The listing builds one solid part. Answer for the finished solid, in the listing's coordinates (mm). Face numbers are marked on the shaded views. A direction names the side the tool comes from. Give positions to 0.01 mm unless a question says otherwise; leave off trailing zeros. Loops run counter-clockwise (first coordinate to the right, second up) from the corner with the lowest first, then second, coordinate; pieces in that order, holes last. Notation, with made-up numbers: M 29.5,29.25 L 60.5,29.25 A16 cw 60.5,51.25 Z; hole C 89,10 d10. An arc over 180 degrees is marked long. Return JSON: item names as keys, results as strings.
from build123d import *

# Parameters (mm, degrees)
F0_W     = 101.6
F0_H     = 101.6
F1_DEPTH = 101.6
F2_R     = 6.35
F3_DEPTH = 101.6
F4_W     = 50.8
F4_H     = 50.8
F5_DEPTH = 50.8


with BuildPart() as f1:
    # F0 (on Front) → F1 (new body)
    with BuildSketch(Plane.XZ):
        with Locations((-50.8, 50.8)):
            Rectangle(F0_W, F0_H)
    extrude(amount=F1_DEPTH)

    # F2 (on face) → F3 (cut)
    with BuildSketch(Plane.XY.offset(101.6)):
        with Locations((-69.063447, -30.745214)):
            Circle(F2_R)
    extrude(amount=-F3_DEPTH, mode=Mode.SUBTRACT)

    # F4 (on face) → F5 (cut)
    with BuildSketch(Plane.XY.offset(101.6)):
        with Locations((-25.4, -25.4)):
            Rectangle(F4_W, F4_H)
    extrude(amount=-F5_DEPTH, mode=Mode.SUBTRACT)


solid = f1.part
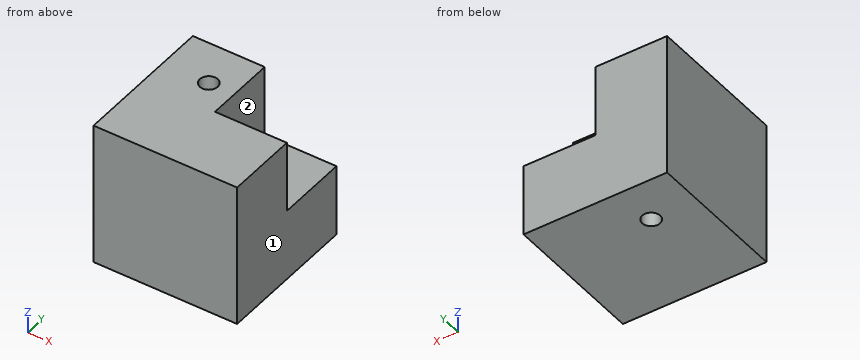
(1) The part is cut by section A-A (x = -71.5). Determine the outline of the cut face in (y, z), and give its area (3 significant figures).
Values follow:
{"outline": "M -101.6,0 L -36.61,0 L -36.61,101.6 L -101.6,101.6 Z; M -24.88,0 L 0,0 L 0,101.6 L -24.88,101.6 Z", "area": "9,130 mm²"}
(2) The part is cut by section C-C (y = -33.5). Determine the outline of the cut face in (x, z).
Values follow:
{"outline": "M -101.6,0 L -74.78,0 L -74.78,101.6 L -101.6,101.6 Z; M -63.34,0 L 0,0 L 0,50.8 L -50.8,50.8 L -50.8,101.6 L -63.34,101.6 Z"}
(3) A tool of negligible diameter and unlimited length cuts with its end or side. For the marked faces 1 and 2, from which of +Z, -Z, +X, -X, +Y, -Y can it reach the whole face along a straight path? Write none if from no direction.
Values follow:
{"face 1": "+Z, -Z, +X, +Y, -Y", "face 2": "+Z, +X, +Y"}
(4) The part is cut by section B-B (y = -13.5). Determine the outline of the cut face in (x, z).
Values follow:
{"outline": "M -101.6,0 L 0,0 L 0,50.8 L -50.8,50.8 L -50.8,101.6 L -101.6,101.6 Z"}
(5) Given pin 1 (12 mm diameter, centred on x = -21, y = -32.5, fed in from +Z), flat-ended and moving along its own axis, determine where the tip first touches the part or whether it passes through.
Values follow:
{"pin 1": "z = 50.8"}
(6) Straight lines are drawn through the part: line 1 along Z through (x, y) = (-41.5, -4.5); line 2 along Y through (x, z) = (-17.5, 89); line 3 along Y through (x, z) = (-66.5, 18.5). For each, find the intervals that lie inside material, in ascending order.
Values follow:
{"line 1": "0 to 50.8", "line 2": "-101.6 to -50.8", "line 3": "-101.6 to -36.55, -24.94 to 0"}
